from build123d import *

# Parameters (mm, degrees)
SKETCH_1_R      = 2
EXTRUDE_1_DEPTH = 3
FILLET_1_R      = 0.3


with BuildPart() as part:
    # 草图1 → 凸台-拉伸1 (new body)
    with BuildSketch(Plane.XY):
        Polygon((1.437729481, -3.151655746), (3.44827868, -0.330717618), (2.010549199, 2.820938127), (-1.437729481, 3.151655746), (-3.44827868, 0.330717618), (-2.010549199, -2.820938127), align=None)
        Circle(SKETCH_1_R, mode=Mode.SUBTRACT)
    extrude(amount=EXTRUDE_1_DEPTH)

    # 圆角1
    fillet_1_edges = [part.edges().sort_by_distance(p)[0] for p in [
        (2.72941394, 1.245110255, 3),
        (0.286409859, 2.986296936, 3),
        (-2.443004081, 1.741186682, 3),
        (-2.72941394, -1.245110255, 3),
        (-0.286409859, -2.986296936, 3),
        (2.443004081, -1.741186682, 3),
    ]]
    fillet(fillet_1_edges, radius=FILLET_1_R)


solid = part.part
Part model, mm, in its own coordinate system. Give positions to 0.01 mm unless a question says otherwise; leave off trailing zeros. Loops run counter-clockwise (first coordinate to the right, second up) from the corner with the lowest first, then second, coordinate; pieces in that order, holes last.
(1) Band-saw the part on A-A (z = 1.3). Write the cut outline in (x, y).
Return value:
outline: (-3.45, 0.33) - (-2.01, -2.82) - (1.44, -3.15) - (3.45, -0.33) - (2.01, 2.82) - (-1.44, 3.15) - close; hole circle Ø4 at (0, 0)
(2) Pull direction Y, two halves, no side cores. Call faces 1 (the cylindrical face through (0, -2, 1)), 2 (the flat face through (-2, -1, 0)), 3 (the cylindrical face through (-2.39, 1.67, 2.91)), 4 (the cylindrical face through (2.39, -1.67, 2.91)): pulls with the +Y half, pulls with the -Y half, needs draft (parallel to the pull), parting line crosses it, or undercut.
Return value:
face 1: undercut
face 2: needs draft
face 3: pulls with the +Y half
face 4: pulls with the -Y half
(3) Drill centre lines: line 1 along Z through (x, y) = (3, -0.5); line 2 along Y through (x, z) = (-1.5, 0.1); line 3 along X through (y, z) = (-0.5, 2.5). Where is each one in solid material? Low to high.
Return value:
line 1: z = 0 to 3
line 2: y = -2.87 to -1.32, 1.32 to 3.06
line 3: x = -3.07 to -1.94, 1.94 to 3.33
